from build123d import *

# Parameters (mm, degrees)
SKETCH1_RX          = 20.32
SKETCH1_RY          = 6.35
SKETCH1_R           = 1.5875
SKETCH1_R_2         = 5.715
BOSS_EXTRUDE1_DEPTH = 3.81
BOSS_EXTRUDE2_START = 3.81
SKETCH1_3_R         = 5.715
BOSS_EXTRUDE2_DEPTH = 3.81
BOSS_EXTRUDE3_START = 3.81
SKETCH1_4_R         = 5.715
BOSS_EXTRUDE3_DEPTH = 11.43


with BuildPart() as part:
    # Sketch1 → Boss-Extrude1 (new body)
    # profile 1 of 3: a face of its own
    with BuildSketch(Plane(origin=(0, 0, 0), x_dir=(1, 0, 0), z_dir=(0, 1, 0))):
        with Locations((0, 0)):
            Ellipse(SKETCH1_RX, SKETCH1_RY)
        with Locations(Location((-15.875, 0, 0), (0, 0, 90))):
            Circle(SKETCH1_R, mode=Mode.SUBTRACT)
        with Locations(Location((15.875, 0, 0), (0, 0, 90))):
            Circle(SKETCH1_R, mode=Mode.SUBTRACT)
        Circle(SKETCH1_R_2, mode=Mode.SUBTRACT)
    # profile 2 of 3: a face of its own
    with BuildSketch(Plane(origin=(0, 0, 0), x_dir=(1, 0, 0), z_dir=(0, 1, 0))):
        Circle(SKETCH1_R_2)
        Polygon((1.466469684, -2.54), (2.932939367, 0), (1.466469684, 2.54), (-1.466469684, 2.54), (-2.932939367, 0), (-1.466469684, -2.54), align=None, mode=Mode.SUBTRACT)
    # profile 3 of 3: a face of its own
    with BuildSketch(Plane(origin=(0, 0, 0), x_dir=(1, 0, 0), z_dir=(0, 1, 0))):
        Polygon((-1.466469684, -2.54), (1.466469684, -2.54), (2.932939367, 0), (1.466469684, 2.54), (-1.466469684, 2.54), (-2.932939367, 0), align=None)
    extrude(amount=BOSS_EXTRUDE1_DEPTH)

    # Sketch1<3> → Boss-Extrude2 (add)
    # profile 1 of 2: a face of its own
    with BuildSketch(Plane(origin=(0, 0, 0), x_dir=(1, 0, 0), z_dir=(0, 1, 0)).offset(BOSS_EXTRUDE2_START)):
        with Locations(Location((0, 0, 0), (0, 0, 90))):
            Circle(SKETCH1_3_R)
        Polygon((1.466469684, -2.54), (2.932939367, 0), (1.466469684, 2.54), (-1.466469684, 2.54), (-2.932939367, 0), (-1.466469684, -2.54), align=None, mode=Mode.SUBTRACT)
    # profile 2 of 2: a face of its own
    with BuildSketch(Plane(origin=(0, 0, 0), x_dir=(1, 0, 0), z_dir=(0, 1, 0)).offset(BOSS_EXTRUDE2_START)):
        Polygon((-1.466469684, -2.54), (1.466469684, -2.54), (2.932939367, 0), (1.466469684, 2.54), (-1.466469684, 2.54), (-2.932939367, 0), align=None)
    extrude(amount=BOSS_EXTRUDE2_DEPTH)

    # Sketch1<4> → Boss-Extrude3 (add)
    with BuildSketch(Plane(origin=(0, 0, 0), x_dir=(1, 0, 0), z_dir=(0, 1, 0)).offset(BOSS_EXTRUDE3_START)):
        with Locations(Location((0, 0, 0), (0, 0, 90))):
            Circle(SKETCH1_4_R)
        Polygon((1.466469684, -2.54), (2.932939367, 0), (1.466469684, 2.54), (-1.466469684, 2.54), (-2.932939367, 0), (-1.466469684, -2.54), align=None, mode=Mode.SUBTRACT)
    extrude(amount=BOSS_EXTRUDE3_DEPTH)


solid = part.part
Read the model definition and answer for the solid it produces. Units are mm, in the model's axes. A direction names the side the tool comes from. Give positions to 0.01 mm unless a question says otherwise; leave off trailing zeros. Loops run counter-clockwise (first coordinate to the right, second up) from the corner with the lowest first, then second, coordinate; pieces in that order, holes last. Notation, with made-up numbers: (-14.75, 49) -> (41.25, 49) arc R23 ccw to (41.25, 67) -> close; hole circle Ø10 at (66, 63.5). An arc over 180 degrees is marked (long way). Use a Markdown table: item, result.
Q1. A tool of negligible diameter and unlimited length cuts with its end or side. For faces 1 (the face through (-14.325, 1.878, 0.344)), 2 (the face through (0, 7.62, 0)), from which of +Z, -Z, +X, -X, +Y, -Y can it reach the whole face along a straight path? Write none if from no direction.
Solved:
| item | result |
|---|---|
| face 1 | +Y, -Y |
| face 2 | +Y |
Q2. Find the intervals of material crossed by line 1 along X through (y, z) = (1.45, 0); line 2 along X through (y, z) = (13.75, 1.25); line 3 along Y through (x, z) = (0, -1), in increasing order.
Solved:
| item | result |
|---|---|
| line 1 | x = -20.32 to -17.46, -14.29 to 14.29, 17.46 to 20.32 |
| line 2 | x = -5.58 to -2.21, 2.21 to 5.58 |
| line 3 | y = 0 to 7.62 |
Q3. Section A-A, the plane y = 11 is taken. Determine the outline of the cut face in (x, z) (3 decimals), then the cut area to 3 significant figures.
Solved:
| item | result |
|---|---|
| outline | circle Ø11.43 at (0, 0); hole (-2.933, 0) -> (-1.466, -2.54) -> (1.466, -2.54) -> (2.933, 0) -> (1.466, 2.54) -> (-1.466, 2.54) -> close |
| area | 80.3 mm^2 |
Q4. Section C-C, the plane y = 4.75 is taken. Determine the outline of the cut face in (x, z) (3 decimals), then the cut area to 3 significant figures.
Solved:
| item | result |
|---|---|
| outline | circle Ø11.43 at (0, 0) |
| area | 103 mm^2 |
Q5. Section B-B, the plane z = -1 is taken. Count the separate pieces of the cut face and the enclosed holes in it, then the cut area to 3 significant figures.
Solved:
| item | result |
|---|---|
| separate pieces | 3 |
| enclosed holes | 0 |
| area | 227 mm^2 |
Q6. Each of these flat-tipped pins is pushed along its axis until it touches: pin 1 (8 mm diameter, centred on x = 5.5, y = 12, fed in from -Z); pin 2 (2.5 mm diameter, centred on x = -0.5, y = 13, fed in from +Z) (3 decimals); pin 3 (1.9 mm diameter, centred on x = 15.875, z = 0, fed in from -Y); pin 4 (1.5 mm diameter, centred on x = 0, y = 10.5, fed in from -Z) (3 decimals). Where does it stop, or does it pass through?
Solved:
| item | result |
|---|---|
| pin 1 | stops at z = -5.51 |
| pin 2 | stops at z = 5.715 |
| pin 3 | passes through |
| pin 4 | stops at z = -5.715 |
Q7. Determine the mould class of faces 3 (the face through (0, 15.24, 3)), 4 (the face through (-5.666, 9.445, 0.744)), 5 (the face through (-2.21, 11.38, 1.25)) for opening direction Z: pulls with the +Z half, pulls with the -Z half, needs draft (parallel to the pull), parting line crosses it, or undercut.
Solved:
| item | result |
|---|---|
| face 3 | needs draft |
| face 4 | parting line crosses it |
| face 5 | undercut |
